Could you check a few things on this model? Use its own coordinates, in mm. Face numbers are marked on the shaded views. A direction names the side the tool comes from. Coordinates: 2 decimals unless noted, no trailing zeros. Order: outer loops, then holes, each group sorted by start corner. A loop starts at its lowest first (then second) coordinate and runs counter-clockwise, first axis right, second up. Notation, with made-up numbers: (50, 76.5) -> (66, 76.5) arc R29 ccw to (66, 110.5) -> close; hole circle Ø5 at (-39, -26). An arc over 180 degrees is marked (long way). Put each result on its own line as item: value. Start each with the question number.
Q1. If we section it at C-C (z = -6.75): Please give me the cut outline in (x, y), and give its area (3 significant figures).
Q2. We'd pull the mould along X, two halves only. Please class the marked faces 4, 5 and 6: +X half, -X half, draft (parallel to the pull), parting line (faces both ways), or undercut.
Q3. If we section it at A-A (z = -9.75): Please give me the cut outline in (x, y), and give its area (3 significant figures).
Q4. Will these pins go through, and if not, where does the flat tip stop? pin 1 (2.5 mm diameter, centred on x = 0, y = -6, fed in from -Z); pin 2 (2 mm diameter, centred on x = 9, y = -4.5, fed in from -Z); pin 3 (1.2 mm diameter, centred on x = 0, y = 4.5, fed in from -Z).
Q5. If we section it at B-B (x = 0): Count the separate pieces of the cut face and the enclosed holes in it, and give its area (3 significant figures).
Q6. For the marked faces 1, 2 and 3, which set-ups out of +Z, -Z, +X, -X, +Y, -Y let a thin tool reach every point of the face, with its end or its side?
Q7. Please list where these lines run through material, in increasing order: line 1 along Z through (x, y) = (5.25, -1.25); line 2 along Z through (x, y) = (10.25, -1); line 3 along Y through (x, z) = (0, -0.95).
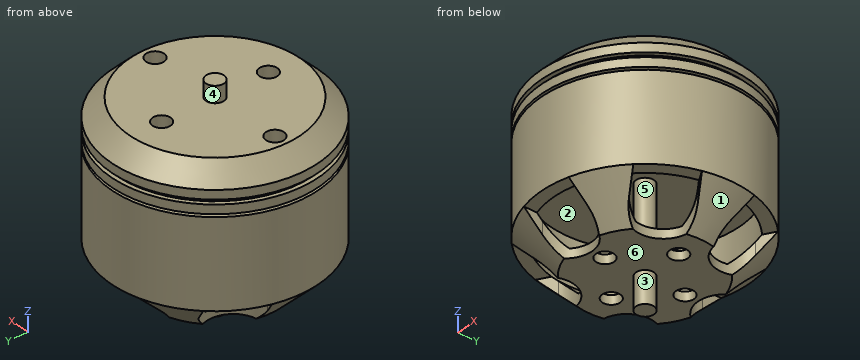
from build123d import *

# Parameters (mm, degrees)
SKETCH3_R          = 1
CUT_EXTRUDE1_DEPTH = 4
SKETCH4_R          = 1
CUT_EXTRUDE2_DEPTH = 3


with BuildPart() as part:
    # Sketch2 → Revolve3 (revolve)
    with BuildSketch(Plane(origin=(0, 0, 0), x_dir=(1, 0, 0), z_dir=(0, 1, 0))):
        Polygon((0, 22), (0, -1.8), (1, -1.8), (1, 0), (9.5, 0), (11.5, 2), (11.5, 3), (11, 3), (11, 3.5), (11.5, 3.5), (11.5, 4.5), (9.5, 4.5), (9.5, 4.8), (11.5, 4.8), (11.5, 14.5), (7.5, 18.5), (1, 18.5), (1, 22), align=None)
        Polygon((2, 17.5), (7.085786438, 17.5), (10.5, 14.085786438), (10.5, 8.994124711), (1, 8.994124711), (1, 16.5), (2, 16.5), align=None, mode=Mode.SUBTRACT)
    revolve(axis=Axis((0, 0, -22), (0, 0, 1)))

    # Sketch3 → Cut-Extrude1 (cut)
    with BuildSketch(Plane(origin=(0, 0, -18.5), x_dir=(-1, 0, 0), z_dir=(0, 0, -1))):
        with Locations((0, 4.5)):
            Circle(SKETCH3_R)
        with Locations((4.5, 0)):
            Circle(SKETCH3_R)
        with Locations((0, -4.5)):
            Circle(SKETCH3_R)
        with Locations((-4.5, 0)):
            Circle(SKETCH3_R)
        with BuildLine():
            Line((-3, 9), (-3, 16.381316394))
            Line((-3, 16.381316394), (3, 16.381316394))
            Line((3, 16.381316394), (3, 9))
            ThreePointArc((3, 9), (0, 6), (-3, 9))
        make_face()
        with BuildLine():
            Line((15.686636144, 5.592581985), (9.294228634, 1.901923789))
            ThreePointArc((9.294228634, 1.901923789), (5.196152423, 3), (6.294228634, 7.098076211))
            Line((6.294228634, 7.098076211), (12.686636144, 10.788734408))
            Line((12.686636144, 10.788734408), (15.686636144, 5.592581985))
        make_face()
        with BuildLine():
            Line((12.686636144, -10.788734408), (6.294228634, -7.098076211))
            ThreePointArc((6.294228634, -7.098076211), (5.196152423, -3), (9.294228634, -1.901923789))
            Line((9.294228634, -1.901923789), (15.686636144, -5.592581985))
            Line((15.686636144, -5.592581985), (12.686636144, -10.788734408))
        make_face()
        with BuildLine():
            Line((-3, -16.381316394), (-3, -9))
            ThreePointArc((-3, -9), (0, -6), (3, -9))
            Line((3, -9), (3, -16.381316394))
            Line((3, -16.381316394), (-3, -16.381316394))
        make_face()
        with BuildLine():
            Line((-15.686636144, -5.592581985), (-9.294228634, -1.901923789))
            ThreePointArc((-9.294228634, -1.901923789), (-5.196152423, -3), (-6.294228634, -7.098076211))
            Line((-6.294228634, -7.098076211), (-12.686636144, -10.788734408))
            Line((-12.686636144, -10.788734408), (-15.686636144, -5.592581985))
        make_face()
        with BuildLine():
            Line((-12.686636144, 10.788734408), (-6.294228634, 7.098076211))
            ThreePointArc((-6.294228634, 7.098076211), (-5.196152423, 3), (-9.294228634, 1.901923789))
            Line((-9.294228634, 1.901923789), (-15.686636144, 5.592581985))
            Line((-15.686636144, 5.592581985), (-12.686636144, 10.788734408))
        make_face()
    extrude(amount=-CUT_EXTRUDE1_DEPTH, mode=Mode.SUBTRACT)

    # Sketch4 → Cut-Extrude2 (cut)
    with BuildSketch(Plane.XY):
        with Locations((0, 6)):
            Circle(SKETCH4_R)
        with Locations((0, -6)):
            Circle(SKETCH4_R)
        with Locations((8, 0)):
            Circle(SKETCH4_R)
        with Locations((-8, 0)):
            Circle(SKETCH4_R)
    extrude(amount=-CUT_EXTRUDE2_DEPTH, mode=Mode.SUBTRACT)


solid = part.part
The answers:
1. outline: circle Ø23 at (0, 0)
1. area: 415 mm^2
2. face 4: parting line
2. face 5: undercut
2. face 6: draft
3. outline: circle Ø23 at (0, 0); circle Ø2 at (0, 0); hole circle Ø21 at (0, 0)
3. area: 72.3 mm^2
4. pin 1: z = -18.5
4. pin 2: z = -14.5
4. pin 3: z = -8.99
5. separate pieces: 3
5. enclosed holes: 0
5. area: 238 mm^2
6. face 1: -Z, +X
6. face 2: none
6. face 3: -Z
7. line 1: -18.5 to -17.5, -8.99 to 0
7. line 2: -15.7 to -14.29, -8.99 to -4.8, -4.5 to -0.8
7. line 3: -10.45 to -7, -5 to 5, 7 to 10.45
